Autodesk Inventor part; units mm, degrees
ref_plane "YZ Plane" through (0, 0, 0) normal (1, 0, 0) x (0, 1, 0)
ref_plane "XZ Plane" through (0, 0, 0) normal (0, 1, 0) x (-1, 0, 0)
ref_plane "XY Plane" through (0, 0, 0) normal (0, 0, 1) x (1, 0, 0)
sketch "Sketch1" plane through (0, 0, 0) normal (0, 1, 0) x (-1, 0, 0)
  line L0 (11.3393, 25.914) -> (-14.0607, 25.914)
  line L1 (-14.0607, 25.914) -> (-14.0607, 13.214)
  line L2 (11.3393, 13.214) -> (11.3393, 25.914)
  arc A0 (-14.0607, 13.214) -> (11.3393, 13.214) centre (-1.3607, 13.214) ccw
  point P0 (0, 0)
  dimension "d1" = 25.4
  dimension "d2" = 25.4
  dimension "d3" = 12.7
  dimension "d4" = 12.7
extrude "Extrusion1" add sketch "Sketch1" along normal blind 25.4
sketch "Sketch2" plane through (0, 25.4, 0) normal (0, 1, 0) x (1, 0, 0)
  arc A0 (14.0607, -13.214) -> (-11.3393, -13.214) centre (1.3607, -13.214) ccw
  circle A1 centre (1.3607, -13.214) radius 2.54
  point P0 (0, 0)
  dimension "d7" = 5.08
extrude "Extrusion2" cut sketch "Sketch2" against normal blind 25.4
properties part number "Hinge"
Work out the finished part from the listing and answer in its coordinate system (mm). Give positions to 0.01 mm unless a question says otherwise; leave off trailing zeros. Order: outer loops, then holes, each group sorted by start corner. A loop starts at its lowest first (then second) coordinate and runs counter-clockwise, first axis right, second up. Notation, with made-up numbers: M 48,-19.5 L 82,-19.5 A29 ccw 82,11.5 Z; hole C -13.75,-12.75 d7. An arc over 180 degrees is marked long. Return JSON: item names as keys, results as strings.
Q1. Find section A-A, the plane y = 3.25. Write down the section's boundary in (x, z), and give its area (3 significant figures).
Answer below:
{"outline": "M -11.34,13.21 A12.7 ccw 14.06,13.21 L 14.06,25.91 L -11.34,25.91 Z; hole C 1.36,13.21 d5.08", "area": "556 mm^2"}
Q2. Find the intervals of material crossed by line 1 along X through (y, z) = (7.25, 13); line 2 along Z through (x, y) = (2, 1.5); line 3 along X through (y, z) = (23.5, 14.5), in increasing order. Write a range as [from, to].
Answer below:
{"line 1": "x = [-11.34, -1.17], [3.89, 14.06]", "line 2": "z = [0.53, 10.76], [15.67, 25.91]", "line 3": "x = [-11.34, -0.83], [3.55, 14.06]"}
Q3. This flat-tipped pin is pushed along its axis until it touches: pin 1 (1 mm diameter, centred on y = 15, z = 4.5, fed in from -X). Where does it stop, or does it pass through?
Answer below:
{"pin 1": "stops at x = -8.33"}
Q4. Find section D-D, the plane x = -5. Write down the section's boundary in (y, z), and give its area (3 significant figures).
Answer below:
{"outline": "M 0,2.22 L 25.4,2.22 L 25.4,25.91 L 0,25.91 Z", "area": "602 mm^2"}
Q5. The mould has two halves that part along Z. Classify faces 1 (the face through (1.081, 12.522, 0.517)), 2 (the face through (2, 25.4, 16)), 3 (the face through (0.81, 12.878, 15.694)): pulls with the +Z half, pulls with the -Z half, needs draft (parallel to the pull), parting line crosses it, or undercut.
Answer below:
{"face 1": "pulls with the -Z half", "face 2": "needs draft", "face 3": "undercut"}
Q6. Find section C-C, the plane z = 15.25. Write down the section's boundary in (x, y), and give its area (3 significant figures).
Answer below:
{"outline": "M -11.34,0 L -0.16,0 L -0.16,25.4 L -11.34,25.4 Z; M 2.88,0 L 14.06,0 L 14.06,25.4 L 2.88,25.4 Z", "area": "568 mm^2"}
Q7. Find section B-B, the plane z = 12.5. Write down the section's boundary in (x, y).
Answer below:
{"outline": "M -11.32,0 L -1.08,0 L -1.08,25.4 L -11.32,25.4 Z; M 3.8,0 L 14.04,0 L 14.04,25.4 L 3.8,25.4 Z"}
